The drawing under review shows one solid part. Ordinate dimensions are in mm from its lowest x, y, z. A direction names the side the tool comes from. Give positions to 0.01 mm unless a question says otherwise; leave off trailing zeros. Order: outer loops, then holes, each group sorted by start corner. A loop starts at its lowest first (then second) coordinate and runs counter-clockwise, first axis right, second up. Notation, with made-up numbers: (27.5, 50) - (58.5, 50) arc R7 ccw to (58.5, 60) - close; hole circle Ø11 at (75, 6). An arc over 180 degrees is marked (long way). Write item = value, one per line. Start each with the question number.
1. We need section B-B, the plane y = 5. Give the boundary of the cut face in (x, z), and give its area (3 significant figures).
2. We need section C-C, the plane x = 2. Give the boundary of the cut face in (y, z).
3. Mouldability with a two-part tool opening along X and no side actions: class the marked faces 3, 4 and 5 as pulls with the +X half, pulls with the -X half, needs draft (parallel to the pull), parting line crosses it, or undercut.
4. Machinability: for the marked faces 1 and 2, which of the approach directions +Z, -Z, +X, -X, +Y, -Y give a long, thin tool a straight path to every point of the face, cutting with its end or side? Answer none if there is none.
5. We need section A-A, the plane z = 6. Give the boundary of the cut face in (x, y), and give its area (3 significant figures).
6. We need section D-D, the plane z = 3.25. Give the boundary of the cut face in (x, y).
7. For P1, Ø1.4, axis at y = 6, z = 9.5, coming from the +X side; P2, Ø3, axis at y = 6, z = 6, coming from the +X side; P3, Ø2, axis at x = 1.5, z = 4, coming from the +Y side; P4, Ø1, axis at x = 6, z = 10.5, coming from the -Y side, all flat-tipped, find the tip position at first contact; note any pin that passes through.
8. Wall thickness on probe 1 along X at (y, z) = (2.5, 5.25); probe 2 along Y at (x, z) = (2.75, 6) (1 decimal); probe 3 along Y at (x, z) = (2, 6.25) (1 decimal): over which ranges is each line inside the solid? List them lowest first.
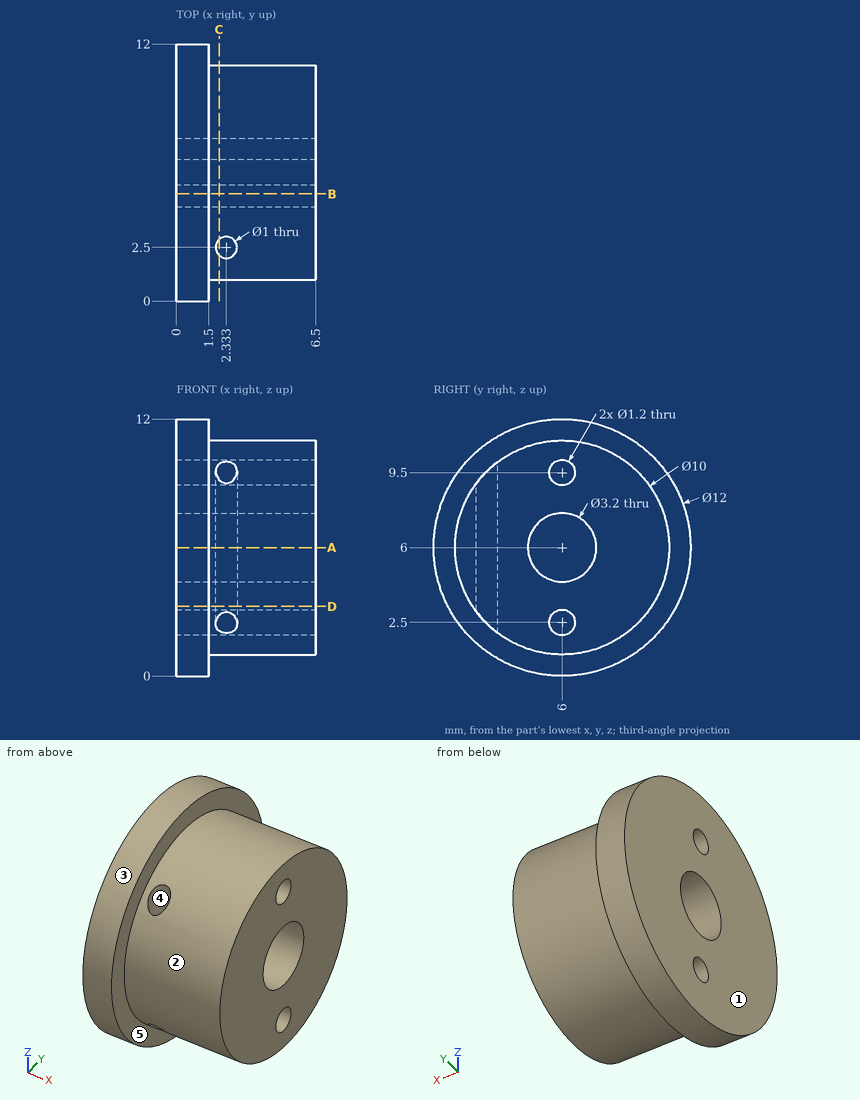
Model answer:
q1.outline = (0, 0.08) - (1.5, 0.08) - (1.5, 1.1) - (6.5, 1.1) - (6.5, 4.75) - (0, 4.75) - close; (0, 7.25) - (6.5, 7.25) - (6.5, 10.9) - (1.5, 10.9) - (1.5, 11.92) - (0, 11.92) - close
q1.area = 50.5 mm2
q2.outline = (2.13, 2.84) - (2.13, 9.16) arc R5 ccw to start; (2.87, 2.1) arc R5 ccw (long way) to (2.87, 9.9) - close; hole circle Ø3.2 at (6, 6); hole circle Ø1.2 at (6, 2.5); hole circle Ø1.2 at (6, 9.5)
q3.face_3 = needs draft
q3.face_4 = undercut
q3.face_5 = pulls with the +X half
q4.face_1 = +Z, -Z, -X, +Y, -Y
q4.face_2 = +X
q5.outline = (0, 0) - (1.5, 0) - (1.5, 1) - (6.5, 1) - (6.5, 4.4) - (0, 4.4) - close; (0, 7.6) - (6.5, 7.6) - (6.5, 11) - (1.5, 11) - (1.5, 12) - (0, 12) - close; hole circle Ø1 at (2.33, 2.5)
q5.area = 46.4 mm2
q6.outline = (0, 0.67) - (1.5, 0.67) - (1.5, 1.82) - (6.5, 1.82) - (6.5, 10.18) - (1.5, 10.18) - (1.5, 11.33) - (0, 11.33) - close; hole circle Ø1 at (2.33, 2.5)
q7.P1 = 6.5
q7.P2 = through
q7.P3 = 11.92
q7.P4 = 3
q8.probe_1 = 0 to 1.83, 2.83 to 6.5
q8.probe_2 = 1 to 2.2, 2.8 to 4.4, 7.6 to 11
q8.probe_3 = 1 to 2.1, 2.9 to 4.4, 7.6 to 11
